Autodesk Inventor part; units mm, degrees
ref_plane "YZ Plane" through (0, 0, 0) normal (1, 0, 0) x (0, 1, 0)
ref_plane "XZ Plane" through (0, 0, 0) normal (0, 1, 0) x (-1, 0, 0)
ref_plane "XY Plane" through (0, 0, 0) normal (0, 0, 1) x (1, 0, 0)
sketch "스케치1" plane through (0, 0, 0) normal (0, 0, 1) x (1, 0, 0)
  circle A0 centre (25.8313, 14.9075) radius 5
  circle A1 centre (18.3313, 22.4075) radius 1.25
  circle A2 centre (18.3313, 7.3526) radius 1.25
  circle A3 centre (33.2769, 22.4075) radius 1.25
  circle A4 centre (46.9521, 27.6627) radius 1.25
  circle A5 centre (46.9521, 2.0974) radius 1.25
  circle A6 centre (33.2769, 7.3526) radius 1.25
  line L0 (25.8041, 29.8443) -> (25.8875, 29.8036)
  line L1 (0, 30) -> (0, 0)
  line L2 (0, 30) -> (51.61, 30)
  line L3 (51.61, 30) -> (51.61, 0)
  line L4 (51.61, 0) -> (0, 0)
  line L5 (0, 0) -> (0, 30)
  circle A7 centre (4.6891, 27.6627) radius 1.25
  circle A8 centre (4.6891, 2.0974) radius 1.25
  dimension "d2" = 10
  dimension "d5" = 2.5
  dimension "d26" = 51.61
extrude "판3" add sketch "스케치1" along normal blind 2
sketch "스케치3" plane through (53.0242, 0, -0.5858) normal (0.7071068, 0, 0.7071068) x (0, 1, 0)
  line L0 (30, 0) -> (0, 0)
  line L1 (0, 0) -> (0, -4.3431)
  line L2 (0, -4.3431) -> (30, -4.3431)
  line L3 (30, -4.3431) -> (30, 0)
edge flange "플랜지2" height 6 angle 45 thickness 2 bend radius 2 thickness toward (0.7071068, 0, 0.7071068) relief tear relief width 2 relief depth 1 corner gap 2 corner form 0 edges at (51.61, 15, 0) (0, 15, 0) wall of the first edge with corners at (53.0242, 30, -0.5858) (53.0242, 0, -0.5858) (56.0953, 0, -3.6569) (56.0953, 30, -3.6569)
bend "절곡부2"
corner "구석2"
sketch "스케치4" plane through (56.6811, 0, -5.0711) normal (1, 0, 0) x (0, 1, 0)
  line L0 (30, 0) -> (0, 0)
  line L1 (0, 0) -> (0, -38.3431)
  line L2 (0, -38.3431) -> (30, -38.3431)
  line L3 (30, -38.3431) -> (30, 0)
edge flange "플랜지3" height 40 angle 45 thickness 2 bend radius 2 thickness toward (1, 0, 0) relief tear relief width 2 relief depth 1 corner gap 2 corner form 0 edges at (56.0953, 15, -3.6569) (-4.4853, 15, -3.6569) wall of the first edge with corners at (56.6811, 30, -5.0711) (56.6811, 0, -5.0711) (56.6811, 0, -43.4142) (56.6811, 30, -43.4142)
bend "절곡부3"
corner "구석3"
sketch "스케치5" plane through (-7.0711, 0, -43.4142) normal (-1, 0, 0) x (0, 0, 1)
  line L0 (0, 30) -> (0, 0)
  circle A0 centre (0, 15) radius 7.5
  circle A1 centre (0, 15) radius 14.969
  line L1 (0, 15) -> (14.969, 15)
  point P0 (43.4142, 0)
  point P1 (0, 7.5)
  point P2 (0, 22.5)
  dimension "d48" = 15
extrude "돌출2" cut sketch "스케치5" against normal blind 66 contours A0 L1 L0 | L1 A0 L0
fillet "모깎기1" radius 2 8 edges at (57.6811, 0, -43.4142) (-6.0711, 0, -43.4142) (-6.0711, 7.5, -43.4142) (-6.0711, 22.5, -43.4142) (-6.0711, 30, -43.4142) (57.6811, 7.5, -43.4142) (57.6811, 22.5, -43.4142) (57.6811, 30, -43.4142)
equation "\"d28\" = BendReliefWidth"
equation "\"d29\" = BendReliefDepth"
equation "\"d30\" = MinimumRemnant"
equation "\"d31\" = TransitionRadius"
equation "\"d34\" = BendRadius"
equation "\"d35\" = CornerReliefSize"
equation "\"d38\" = BendReliefWidth"
equation "\"d39\" = BendReliefDepth"
equation "\"d40\" = MinimumRemnant"
equation "\"d41\" = TransitionRadius"
equation "\"d44\" = BendRadius"
equation "\"d45\" = CornerReliefSize"
equation "\"TransitionRadius\" = BendRadius"
properties part number "motor_u" material "알루미늄 6061"
Design review of the part built by this model. Coordinates are the model's own, in mm. A direction names the side the tool comes from. Coordinates: 2 decimals unless noted, no trailing zeros. Loops run counter-clockwise (first coordinate to the right, second up) from the corner with the lowest first, then second, coordinate; pieces in that order, holes last. Notation, with made-up numbers: (87.25, 47.5) -> (116.25, 47.5) arc R20 ccw to (116.25, 62.5) -> close; hole circle Ø2 at (35, 39.25). An arc over 180 degrees is marked (long way). Use a Markdown table: item, result. Add a question column.
Item 1: Wall thickness on L1, parallel to X at y = 14.25, z = -23; L2, parallel to Z at x = 10.5, y = 1; L3, parallel to X at y = 1.5, z = -1.5: over which ranges is each line inside the solid? List them lowest first. Write a range as from..to.
Item 2: The part is to be moulded in two halves that separate along Y. For faces 1 (the cylindrical face through (24.75, 19.79, 0.99)), 2 (the cylindrical face through (-0.78, 15.21, -0.16)), 3 (the cylindrical face through (-6.09, 29.43, -42.81)), say which applies: +Y half, -Y half, draft (parallel to the pull), parting line (faces both ways), or undercut.
Item 3: We need section D-D, the plane z = -39. Write out the cut boundary in (x, y), and give its area (3 significant figures).
Item 4: We need section C-C, the plane y = 5. Write out the cut boundary in (x, z).
Item 5: Machinability: for faces 4 (the cylindrical face through (-4.923, 15.21, -4.316)), 5 (the flat face through (58.681, 15, -25)), which of the approach directions +Z, -Z, +X, -X, +Y, -Y give a long, thin tool a straight path to every point of the face, cutting with its end or side? Answer none if there is none.
Item 6: Clearance check with flat-ended pins moving along their axes: P1, Ø6, axis at x = 25.83, y = 14.91, coming from the +Z side; P2, Ø3, axis at x = 46.95, y = 27.66, coming from the +Z side; P3, Ø2, axis at x = 18.5, y = 17.5, coming from the -Z side. State where each tip first meets the part, or that it passes through.
Item 7: We need section B-B, the plane y = 16.75. Write out the cut boundary in (x, z).
Item 8: We need section A-A, the plane z = -32. Write out the cut boundary in (x, y).
Numbers:
| question | item | result |
|---|---|---|
| 1 | L1 | x = -7.07..-5.07, 56.68..58.68 |
| 1 | L2 | z = 0..2 |
| 1 | L3 | x = -5.16..-2.33, 53.94..56.77 |
| 2 | face 1 | undercut |
| 2 | face 2 | draft |
| 2 | face 3 | +Y half |
| 3 | outline | (-7.07, 0) -> (-5.07, 0) -> (-5.07, 8.94) -> (-7.07, 8.94) -> close; (-7.07, 21.06) -> (-5.07, 21.06) -> (-5.07, 30) -> (-7.07, 30) -> close; (56.68, 0) -> (58.68, 0) -> (58.68, 8.94) -> (56.68, 8.94) -> close; (56.68, 21.06) -> (58.68, 21.06) -> (58.68, 30) -> (56.68, 30) -> close |
| 3 | area | 71.5 mm^2 |
| 4 | outline | (-7.07, -43.41) -> (-5.07, -43.41) -> (-5.07, -5.07) arc R2 cw to (-4.49, -3.66) -> (-1.41, -0.59) arc R2 cw to (0, 0) -> (51.61, 0) arc R2 cw to (53.02, -0.59) -> (56.1, -3.66) arc R2 cw to (56.68, -5.07) -> (56.68, -43.41) -> (58.68, -43.41) -> (58.68, -5.07) arc R4 ccw to (57.51, -2.24) -> (54.44, 0.83) arc R4 ccw to (51.61, 2) -> (0, 2) arc R4 ccw to (-2.83, 0.83) -> (-5.9, -2.24) arc R4 ccw to (-7.07, -5.07) -> close |
| 5 | face 4 | -Z, +Y, -Y |
| 5 | face 5 | +Z, -Z, +X, +Y, -Y |
| 6 | P1 | passes through |
| 6 | P2 | stops at z = 2 |
| 6 | P3 | stops at z = 0 |
| 7 | outline | (-7.07, -36.12) -> (-5.07, -36.12) -> (-5.07, -5.07) arc R2 cw to (-4.49, -3.66) -> (-1.41, -0.59) arc R2 cw to (0, 0) -> (21.18, 0) -> (21.18, 2) -> (0, 2) arc R4 ccw to (-2.83, 0.83) -> (-5.9, -2.24) arc R4 ccw to (-7.07, -5.07) -> close; (30.48, 0) -> (51.61, 0) arc R2 cw to (53.02, -0.59) -> (56.1, -3.66) arc R2 cw to (56.68, -5.07) -> (56.68, -36.12) -> (58.68, -36.12) -> (58.68, -5.07) arc R4 ccw to (57.51, -2.24) -> (54.44, 0.83) arc R4 ccw to (51.61, 2) -> (30.48, 2) -> close |
| 8 | outline | (-7.07, 0) -> (-5.07, 0) -> (-5.07, 30) -> (-7.07, 30) -> close; (56.68, 0) -> (58.68, 0) -> (58.68, 30) -> (56.68, 30) -> close |
